Geometry: final body of the model. Coordinates: model frame, mm. A direction names the side the tool comes from. Give positions to 0.01 mm unless a question says otherwise; leave off trailing zeros. Order: outer loops, then holes, each group sorted by start corner. A loop starts at its lowest first (then second) coordinate and runs counter-clockwise, first axis right, second up. Notation, with made-up numbers: (82, -3.75) -> (137, -3.75) arc R30 ccw to (137, 30.25) -> close; hole circle Ø1 at (15, 3.25). An arc over 180 degrees is marked (long way). One line per item, written item: value. Start each with the question number.
```python
from build123d import *

# Parameters (mm, degrees)
F0_R      = 29.25
F1_DEPTH  = 25
F2_R      = 29.25
F3_DEPTH  = 10
F4_DEPTH  = 10
F9_R      = 8.5
F10_DEPTH = 152
F11_ANGLE = 180


with BuildPart() as f1:
    # F0 (on Top) → F1 (new body)
    with BuildSketch(Plane.XY):
        Circle(F0_R)
    extrude(amount=F1_DEPTH)

    # F2 (on face) → F3 (join)
    with BuildSketch(Plane.XY.offset(25)):
        with BuildLine():
            Line((28.24251, 37.508036), (11.563291, 37.508036))
            ThreePointArc((11.563291, 37.508036), (0.845642, 39.240889), (-9.936709, 37.971362))
            Line((-9.936709, 37.971362), (-28.076276, 37.971362))
            Line((-28.076276, 37.971362), (-36.944126, 13.254964))
            ThreePointArc((-36.944126, 13.254964), (0, -39.25), (36.944126, 13.254964))
            Line((36.944126, 13.254964), (28.24251, 37.508036))
        make_face()
        Circle(F2_R, mode=Mode.SUBTRACT)
        Circle(F2_R)
    extrude(amount=F3_DEPTH)

    # F2 (on face) → F4 (join, symmetric)
    with BuildSketch(Plane.XY.offset(25)):
        Polygon((11.563291, 61.137354), (11.563291, 37.508036), (28.24251, 37.508036), (19.764687, 61.137354), align=None)
        Polygon((-28.076276, 37.971362), (-9.936709, 37.971362), (-9.936709, 61.137354), (-19.764687, 61.137354), align=None)
    extrude(amount=F4_DEPTH, both=True)

    # F9 (on face) → F10 (cut)
    with BuildSketch(Plane(origin=(0, 34.499137, 59.754259), x_dir=(1, 0, 0), z_dir=(0, 0.5, 0.866025))):
        with Locations((0, -20.857124)):
            Circle(F9_R)
    extrude(amount=-F10_DEPTH, mode=Mode.SUBTRACT)


with BuildPart() as f1_1:
    # F11: moved
    add(f1.part.rotate(Axis((24.003598, 49.322695, 15), (0.337706, -0.941252, 0)), F11_ANGLE))


solid = f1_1.part
```
1. Cut plane C-C, the plane y = 71. Return loops of the section in (x, z), then the cut area to 3 significant figures.
2. Cut plane B-B, the plane z = 10. State how many separate pieces and enclosed holes the cut face has, then the cut area to 3 significant figures.
3. Cut plane D-D, the plane x = 34. Return loops of the section in (y, z), then the cut area to 3 significant figures.
4. Pin query (flat end, axial travel): P1, Ø6, axis at x = 77.5, z = 4, coming from the +Y side; P2, Ø17, axis at x = 30.5, y = 54, coming from the +Z side; P3, Ø2, axis at x = 55.5, z = 26, coming from the +Y side; P4, Ø8, axis at y = 57.5, z = 8.5, coming from the -X side. Return the tip coordinate at first contact, or that it passes through.
5. Material intervals for L1, parallel to Z at x = 104, y = 33.5; L2, parallel to X at y = 13, z = 8; L3, parallel to Y at x = 87, z = 22, sorted ascending. Write a range as [from, to].
6. Draft query along Y for faces 6 (the flat face through (74, 27, 30)), 7 (the cylindrical face through (99.64, -3.11, 0.07)), 8 (the flat face through (22.89, 63.71, 5.14)), 9 (the flat face through (50.16, 70.95, 4.86)). Return one class per face: pulls with the +Y half, pulls with the -Y half, needs draft (parallel to the pull), parting line crosses it, or undercut.
7. Cut plane A-A, the plane x = 49. Return loops of the section in (y, z).
8. Access query for faces 1 (the flat face through (64.518, 67.984, 9.93)), 2 (the flat face through (33.5, 57.36, 5.14)), 3 (the flat face through (34.77, 42.884, 10.07)), 4 (the flat face through (29, 53, 15)), 5 (the cylindrical face through (46.07, 35.55, 17.68)). Directions: +Z, -Z, +X, -X, +Y, -Y. A direction counts if a zero-diameter tool reaches every point of the face in a straight line with its end or side. Return the directions, or none.
Answers follow:
1. outline: (50.12, -5) -> (75.9, -5) -> (75.9, 5) -> (68.18, 5) -> (68.18, 15) -> (50.12, 15) -> close
1. area: 438 mm²
2. separate pieces: 3
2. enclosed holes: 1
2. area: 3,040 mm²
3. outline: (21.46, -5) -> (56.75, -5) -> (56.75, 15) -> (42.25, 15) -> (42.25, 5) -> (21.46, 5) -> close
3. area: 498 mm²
4. P1: stops at y = 71.83
4. P2: stops at z = 15
4. P3: stops at y = 50.03
4. P4: stops at x = 19.76
5. L1: z = [-5, 5]
5. L2: x = [47.95, 74.04], [89.49, 99.83]
5. L3: y = [0.36, 2.2], [20.56, 52.66]
6. face 6: needs draft
6. face 7: parting line crosses it
6. face 8: pulls with the +Y half
6. face 9: undercut
7. outline: (-3.84, -5) -> (56.86, -5) -> (56.86, 5) -> (41.88, 5) -> (41.88, 30) -> (11.14, 30) -> (11.14, 5) -> (-3.84, 5) -> close; (72.36, -5) -> (85.22, -5) -> (85.22, 15) -> (72.36, 15) -> close
8. face 1: +Z, +X
8. face 2: +Z, -Z, +Y
8. face 3: +Z, -Y
8. face 4: +Z, -X, +Y, -Y
8. face 5: +Z
